```python
from build123d import *

# Parameters (mm, degrees)
SKETCH_1_W          = 70
SKETCH_1_H          = 60
SKETCH_1_R          = 1.6
EXTRUDE_1_DEPTH     = 3
EXTRUDE_2_DEPTH     = 3
FILLET_1_R          = 10
FILLET_3_R          = 10
SKETCH_4_R          = 3.1
CUT_EXTRUDE_1_DEPTH = 10
SKETCH_5_R          = 2.5
CUT_EXTRUDE_2_DEPTH = 156.311257048


with BuildPart() as part:
    # 草图1 → 凸台-拉伸1 (new body)
    with BuildSketch(Plane(origin=(0, 0, 0), x_dir=(1, 0, 0), z_dir=(0, 1, 0))):
        with Locations((25, 25)):
            Rectangle(SKETCH_1_W, SKETCH_1_H)
        with Locations(Location((0, 50, 0), (0, 0, 270))):
            Circle(SKETCH_1_R, mode=Mode.SUBTRACT)
        with Locations(Location((50, 50, 0), (0, 0, 90))):
            Circle(SKETCH_1_R, mode=Mode.SUBTRACT)
        with Locations(Location((50, 0, 0), (0, 0, 270))):
            Circle(SKETCH_1_R, mode=Mode.SUBTRACT)
        with Locations(Location((0, 0, 0), (0, 0, 90))):
            Circle(SKETCH_1_R, mode=Mode.SUBTRACT)
    extrude(amount=EXTRUDE_1_DEPTH)

    # 草图2 → 凸台-拉伸2 (add)
    with BuildSketch(Plane(origin=(0, 0, 0), x_dir=(1, 0, 0), z_dir=(0, 1, 0))):
        Polygon((-10, -5), (60, -5), (60, -25), (-3.639610307, -88.639610307), (-58.172444533, -88.639610307), (-141.639610307, -88.639610307), (-98, -45), (-10, -45), align=None)
    extrude(amount=EXTRUDE_2_DEPTH)

    # 圆角1
    fillet_1_edges = [part.edges().sort_by_distance(p)[0] for p in [
        (-10, 1.5, 45),
        (-3.639610307, 1.5, 88.639610307),
        (60, 1.5, 25),
        (-10, 1.5, -55),
        (60, 1.5, -55),
    ]]
    fillet(fillet_1_edges, radius=FILLET_1_R)

    # 圆角3
    fillet_3_edges = [part.edges().sort_by_distance(p)[0] for p in [
        (-98, 1.5, 45),
        (-141.639610307, 1.5, 88.639610307),
    ]]
    fillet(fillet_3_edges, radius=FILLET_3_R)

    # 草图4 → 切除-拉伸1 (cut)
    with BuildSketch(Plane(origin=(0, 3, 0), x_dir=(1, 0, 0), z_dir=(0, 1, 0))):
        with Locations(Location((-117.497474683, -78.639610307, 0), (0, 0, 270))):
            Circle(SKETCH_4_R)
    extrude(amount=-CUT_EXTRUDE_1_DEPTH, mode=Mode.SUBTRACT)

    # 草图5 → 切除-拉伸2 (cut, through all)
    with BuildSketch(Plane(origin=(0, 3, 0), x_dir=(1, 0, 0), z_dir=(0, 1, 0))):
        with Locations(Location((20, -10, 0), (0, 0, 270))):
            Circle(SKETCH_5_R)
        with Locations(Location((30, -10, 0), (0, 0, 90))):
            Circle(SKETCH_5_R)
        with BuildLine():
            Line((11, 30), (20, 30))
            Line((20, 30), (20, 39))
            ThreePointArc((20, 39), (25, 44), (30, 39))
            Line((30, 39), (30, 30))
            Line((30, 30), (39, 30))
            ThreePointArc((39, 30), (44, 25), (39, 20))
            Line((39, 20), (30, 20))
            Line((30, 20), (30, 11))
            ThreePointArc((30, 11), (25, 6), (20, 11))
            Line((20, 11), (20, 20))
            Line((20, 20), (11, 20))
            ThreePointArc((11, 20), (6, 25), (11, 30))
        make_face()
    extrude(amount=-CUT_EXTRUDE_2_DEPTH, mode=Mode.SUBTRACT)


solid = part.part
```
For this review, take the finished solid that the model builds, in its own axes (mm). A direction names the side the tool comes from. Coordinates: 2 decimals unless noted, no trailing zeros. Loops run counter-clockwise (first coordinate to the right, second up) from the corner with the lowest first, then second, coordinate; pieces in that order, holes last. Notation, with made-up numbers: (-24, -9) - (-3, -9) arc R25 cw to (-3, 27) - close; hole circle Ø5 at (25.5, 5). An arc over 180 degrees is marked (long way). Use one line per item in the form item = value. Start each with the question number.
1) Take a section at C-C (z = -25). State the section outline as (x, y) points.
2) For faces 1 (the face through (25, 2, -6)), 2 (the face through (-126.67, 1.52, 82.62)), list the 3-axis set-ups (+Z, -Z, +X, -X, +Y, -Y) from which the entire face can be reached by the end or side of a thin tool; tool diameter is ignored.
3) Take a section at D-D (y = 1.45). State how many separate pieces and enclosed holes the cut face has, plus the area to 3 significant figures.
4) Draft analysis for pull direction Z (two halves, no side actions). For faces 3 (the face through (-118.685, 1.521, 81.503)), 4 (the face through (-12, 0, 48)), 5 (the face through (29, 1, 56)), 6 (the face through (-12.85, 1.52, 41.99)), state which applies: released by +Z, released by -Z, zero draft, split by the parting line, or undercut.
5) Take a section at A-A (x = 25). State the section outline as (y, z) points, plus the area to 3 significant figures.
6) To check wall thickness, follow probe 1 along X at (y, z) = (2.2, 10); probe 2 along X at (y, z) = (1.45, 0); probe 3 along Z at (x, y) = (-37, 1.85). State the ranges of each line that lie inside material, in increasing order. Write a range as from..to.
7) Take a section at B-B (z = 10). State the section outline as (x, y) points.
8) For pin 1 (6 mm diameter, centred on x = -71, z = 65.5, fed in from -Y); pin 2 (1.5 mm diameter, centred on x = 36.5, y = 2, fed in from +Z); pin 3 (1.5 mm diameter, centred on y = 1.5, z = -17, fed in from -X), all flat-tipped, find the tip position at first contact; note any pin that passes through.
From the geometry:
q1.outline = (-10, 0) - (6, 0) - (6, 3) - (-10, 3) - close; (44, 0) - (60, 0) - (60, 3) - (44, 3) - close
q2.face_1 = +Y, -Y
q2.face_2 = -X, +Y, -Y
q3.separate_pieces = 1
q3.enclosed_holes = 8
q3.area = 12,000 mm2
q4.face_3 = undercut
q4.face_4 = zero draft
q4.face_5 = released by +Z
q4.face_6 = released by -Z
q5.outline = (0, -55) - (3, -55) - (3, -44) - (0, -44) - close; (0, -6) - (3, -6) - (3, 60) - (0, 60) - close
q5.area = 231 mm2
q6.probe_1 = -10..17.5, 22.5..27.5, 32.5..60
q6.probe_2 = -10..-1.6, 1.6..48.4, 51.6..60
q6.probe_3 = 45..88.64
q7.outline = (-10, 0) - (17.5, 0) - (17.5, 3) - (-10, 3) - close; (22.5, 0) - (27.5, 0) - (27.5, 3) - (22.5, 3) - close; (32.5, 0) - (60, 0) - (60, 3) - (32.5, 3) - close
q8.pin_1 = 0
q8.pin_2 = 49.25
q8.pin_3 = -10
